```python
from build123d import *

# Parameters (mm, degrees)
SKETCH1_W           = 120
SKETCH1_H           = 92
BOSS_EXTRUDE1_DEPTH = 1
SKETCH2_W           = 1
SKETCH2_H           = 92
BOSS_EXTRUDE2_DEPTH = 23
FILLET1_R           = 3
FILLET2_R           = 3
FILLET3_R           = 3


with BuildPart() as part:
    # Sketch1 → Boss-Extrude1 (new body)
    with BuildSketch(Plane.XY):
        Rectangle(SKETCH1_W, SKETCH1_H)
    extrude(amount=BOSS_EXTRUDE1_DEPTH)

    # Sketch2 → Boss-Extrude2 (add)
    with BuildSketch(Plane.XY.offset(1)):
        with Locations((-59.5, 0)):
            Rectangle(SKETCH2_W, SKETCH2_H)
    boss_extrude2 = extrude(amount=BOSS_EXTRUDE2_DEPTH)

    # Fillet1
    fillet1_edges = [part.edges().sort_by_distance(p)[0] for p in [
        (-60, 0, 0),
    ]]
    fillet(fillet1_edges, radius=FILLET1_R)

    # Fillet2
    fillet2_edges = [part.edges().sort_by_distance(p)[0] for p in [
        (-59, 0, 1),
    ]]
    fillet(fillet2_edges, radius=FILLET2_R)

    # Mirror3: Boss-Extrude2 across plane
    add(boss_extrude2.mirror(Plane(origin=(0, 0, 0), x_dir=(0, 0, 1), z_dir=(1, 0, 0))))

    # Fillet3
    fillet3_edges = [part.edges().sort_by_distance(p)[0] for p in [
        (59, 0, 1),
        (60, 0, 0),
    ]]
    fillet(fillet3_edges, radius=FILLET3_R)


solid = part.part
```
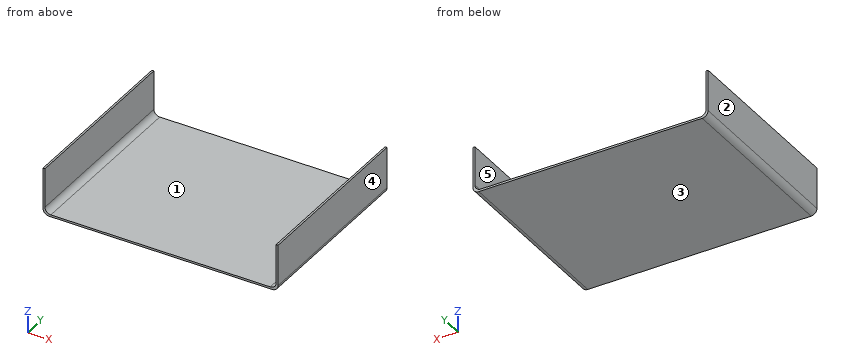
Verification items for the finished model (mm, model axes). Face numbers are marked on the shaded views. A direction names the side the tool comes from. Coordinates: 2 decimals unless noted, no trailing zeros. Write each loop counter-clockwise with the first axis right and the second up, starting at its lowest first coordinate (ties: lowest second). Pieces come first, ordered by that corner, then holes. Notation, with made-up numbers: M -10.5,63.25 L 8.5,63.25 A17 ccw 8.5,92.25 Z; hole C 4,78.25 d10. An arc over 180 degrees is marked long. Answer as a JSON object with one key per item and string values. Group by question number.
(1) Tool access check on the marked faces 4 and 5. Record the directions out of +Z, -Z, +X, -X, +Y, -Y that give a thin tool (end or side, any length) a straight path to the whole face; none if there is none.
(2) Release check for a two-part mould opening along X. For the marked faces 1, 2 and 3 record: +X half, -X half, draft (parallel to the pull), parting line (faces both ways), or undercut.
(3) Cross-section at A-A, the plane z = 17. Record the cut outline in (x, y), and give its area (3 significant figures).
(4) Cross-section at C-C, the plane x = 16.5. Record the cut outline in (y, z).
(5) Cross-section at B-B, the plane y = -0.5. Record the cut outline in (x, z), and give its area (3 significant figures).
(6) Material ranges on line 1 (X direction, y = -23.5, z = 9.75); line 2 (Z direction, x = 52.5, y = 3.5); line 3 (X direction, y = 40, z = 2.25), recorded low to high.
(7) Gauge pin test, flat ends, axial feed: pin 1 (10 mm diameter, centred on x = 30.5, y = 8, fed in from +Z); pin 2 (12 mm diameter, centred on x = -26.5, z = 10.5, fed in from +Y). Record the tip position at first contact, or that the pin passes through.
Reply:
{
 "1": {"face 4": "+Z, -Z, +X, +Y, -Y", "face 5": "+Z, +Y, -Y"},
 "2": {"face 1": "undercut", "face 2": "-X half", "face 3": "draft"},
 "3": {"outline": "M -60,-46 L -59,-46 L -59,46 L -60,46 Z; M 59,-46 L 60,-46 L 60,46 L 59,46 Z", "area": "184 mm²"},
 "4": {"outline": "M -46,0 L 46,0 L 46,1 L -46,1 Z"},
 "5": {"outline": "M -60,3 A3 ccw -57,0 L 57,0 A3 ccw 60,3 L 60,24 L 59,24 L 59,4 A3 cw 56,1 L -56,1 A3 cw -59,4 L -59,24 L -60,24 Z", "area": "166 mm²"},
 "6": {"line 1": "-60 to -59, 59 to 60", "line 2": "0 to 1", "line 3": "-59.9 to -58.44, 58.44 to 59.9"},
 "7": {"pin 1": "z = 1", "pin 2": "through"}
}
